Build history of the part. All positions in model axes, mm. A direction names the side the tool comes from. Coordinates: 2 decimals unless noted, no trailing zeros. Write each loop counter-clockwise with the first axis right and the second up, starting at its lowest first coordinate (ties: lowest second). Pieces come first, ordered by that corner, then holes.
```python
from build123d import *

# Parameters (mm, degrees)
SKETCH1_R           = 75
BOSS_EXTRUDE1_DEPTH = 250
CUT_EXTRUDE1_START  = 100
SKETCH2_R           = 12.5
CUT_EXTRUDE1_DEPTH  = 33


with BuildPart() as part:
    # Sketch1 → Boss-Extrude1 (new body)
    with BuildSketch(Plane.XY):
        with BuildLine():
            Line((-325, 132), (325, 132))
            Line((325, 132), (325, 100))
            Line((325, 100), (156, 100))
            ThreePointArc((156, 100), (120.644660941, 85.355339059), (106, 50))
            Line((106, 50), (106, 0))
            ThreePointArc((106, 0), (0, -106), (-106, 0))
            Line((-106, 0), (-106, 50))
            ThreePointArc((-106, 50), (-120.644660941, 85.355339059), (-156, 100))
            Line((-156, 100), (-325, 100))
            Line((-325, 100), (-325, 132))
        make_face()
        Circle(SKETCH1_R, mode=Mode.SUBTRACT)
    extrude(amount=BOSS_EXTRUDE1_DEPTH)

    # Sketch2 → Cut-Extrude1 (cut, through all)
    with BuildSketch(Plane(origin=(0, 0, 0), x_dir=(1, 0, 0), z_dir=(0, 1, 0)).offset(CUT_EXTRUDE1_START)):
        with Locations((-250, -62.5)):
            Circle(SKETCH2_R)
        with Locations((250, -62.5)):
            Circle(SKETCH2_R)
        with Locations((250, -187.5)):
            Circle(SKETCH2_R)
        with Locations((-250, -187.5)):
            Circle(SKETCH2_R)
    extrude(amount=CUT_EXTRUDE1_DEPTH, mode=Mode.SUBTRACT)


solid = part.part
```
1. Flat gauge pins, fed straight in: pin 1 (25 mm diameter, centred on y = 32.5, z = 128.5, fed in from -X); pin 2 (5 mm diameter, centred on y = -63, z = 67, fed in from +X); pin 3 (15 mm diameter, centred on x = -250, z = 62.5, fed in from +Y); pin 4 (10 mm diameter, centred on y = -66.5, z = 190.5, fed in from -X). Where does each tip first touch, or does it go through?
Computed values:
pin 1: stops at x = -106
pin 2: stops at x = 87.04
pin 3: passes through
pin 4: stops at x = -86.34
2. Probe line 1 along X through (y, z) = (124, 187.5); line 2 along Z through (x, y) = (250, 115); line 3 along Y through (x, z) = (0, 90). List the from-to ranges inside material, lowest first.
Computed values:
line 1: x = -325 to -262.5, -237.5 to 237.5, 262.5 to 325
line 2: z = 0 to 50, 75 to 175, 200 to 250
line 3: y = -106 to -75, 75 to 132
3. 3-axis set-ups, long thin cutter, end or side, ignore diameter. For faces 4 (the face through (-106, 25, 123)), 5 (the face through (2, 84, 0)), 6 (the face through (242, 100, 123)): which of +Z, -Z, +X, -X, +Y, -Y reach the whole face in a straight line?
Computed values:
face 4: +Z, -Z, -X, -Y
face 5: -Z, +X, -X, +Y, -Y
face 6: +Z, -Z, +X, -Y
4. Saw through at B-B on x = -250. List the corners of the cut face in (y, z), plus the area to 3 significant figures.
Computed values:
outline: (100, 0) - (132, 0) - (132, 50) - (100, 50) - close; (100, 75) - (132, 75) - (132, 175) - (100, 175) - close; (100, 200) - (132, 200) - (132, 250) - (100, 250) - close
area: 6,400 mm2
5. Mould opens along X. For faces 1 (the face through (262, 116, 184)), 2 (the face through (325, 116, 123)), 3 (the face through (-120.258, 84.964, 123.25)) say: +X half, -X half, draft (parallel to the pull), parting line (faces both ways), or undercut.
Computed values:
face 1: undercut
face 2: +X half
face 3: -X half
6. Saw through at C-C on z = 29. List the corners of the cut face in (x, y).
Computed values:
outline: (-325, 100) - (-156, 100) arc R50 cw to (-106, 50) - (-106, 0) arc R106 ccw to (106, 0) - (106, 50) arc R50 cw to (156, 100) - (325, 100) - (325, 132) - (-325, 132) - close; hole circle Ø150 at (0, 0)
7. Saw through at A-A on z = 62.5. List the corners of the cut face in (x, y), plus the area to 3 significant figures.
Computed values:
outline: (-325, 100) - (-262.5, 100) - (-262.5, 132) - (-325, 132) - close; (-237.5, 100) - (-156, 100) arc R50 cw to (-106, 50) - (-106, 0) arc R106 ccw to (106, 0) - (106, 50) arc R50 cw to (156, 100) - (237.5, 100) - (237.5, 132) - (-237.5, 132) - close; (262.5, 100) - (325, 100) - (325, 132) - (262.5, 132) - close; hole circle Ø150 at (0, 0)
area: 41,500 mm2
8. Saw through at D-D on x = 0. List the corners of the cut face in (y, z), plus the area to 3 significant figures.
Computed values:
outline: (-106, 0) - (-75, 0) - (-75, 250) - (-106, 250) - close; (75, 0) - (132, 0) - (132, 250) - (75, 250) - close
area: 22,000 mm2
